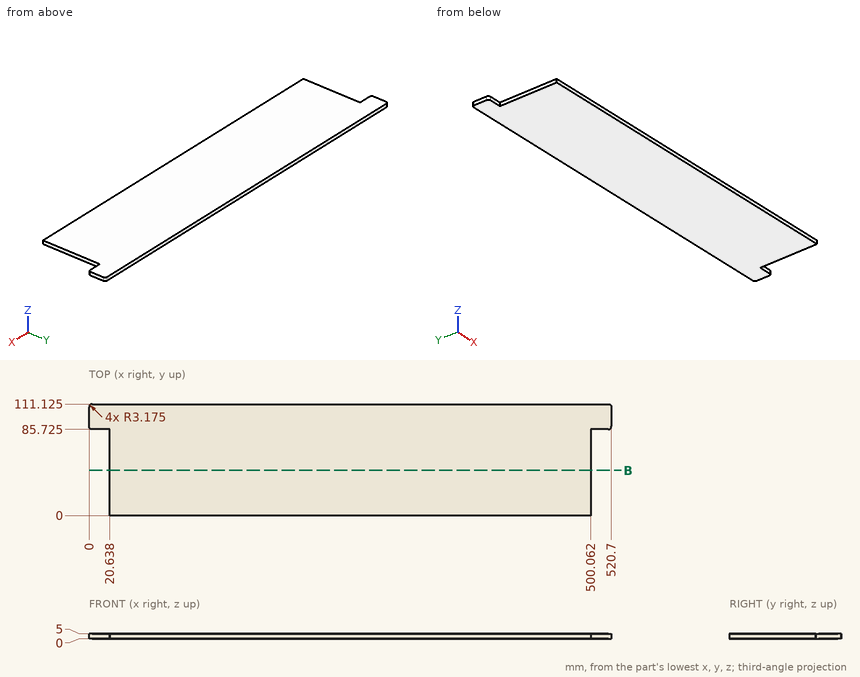
Here's the drawing with two shaded views (mm, measured from the low corner). I have some questions. Give positions to 0.01 mm unless a question says otherwise; leave off trailing zeros. Loops run counter-clockwise (first coordinate to the right, second up) from the corner with the lowest first, then second, coordinate; pieces in that order, holes last. Notation, with made-up numbers: M 39,6.25 L 81,6.25 A32 ccw 81,32.25 Z; hole C -32.75,0.25 d10. An arc over 180 degrees is marked long. One line per item, written item: value.
1) Please list where these lines run through material, in increasing order: line 1 (X direction, y = 54, z = 0.85); line 2 (X direction, y = 87, z = 3.3).
Geometry check:
line 1: x = 20.64 to 500.06
line 2: x = 0.63 to 520.07
2) I'm going to push flat-ended pins straight in: pin 1 (2 mm diameter, centred on x = 451.5, z = 2.5, fed in from -Y); pin 2 (2.5 mm diameter, centred on y = 21.5, z = 2, fed in from +X). Where does each tip first touch, or does it pass through?
Geometry check:
pin 1: stops at y = 0
pin 2: stops at x = 500.06
3) Imagine slicing it at B-B on y = 45. Write out the boundary of the cut face in (x, z).
Geometry check:
outline: M 20.64,0 L 500.06,0 L 500.06,5 L 20.64,5 Z
